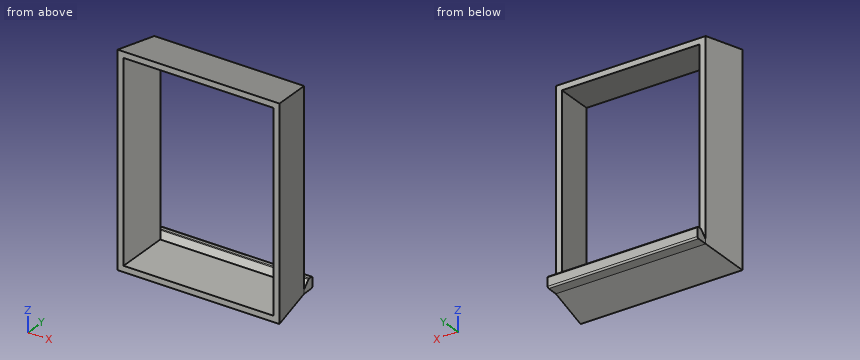
from build123d import *

# Parameters (mm, degrees)
BOSS_EXTRUDE1_DEPTH = 20
LOFT1_START         = -34.8
LOFT1_DEPTH         = 69.6
LOFT1_START_2       = -28
LOFT1_2_DEPTH       = 56
BOSS_EXTRUDE2_START = -2
BOSS_EXTRUDE2_DEPTH = 50
BOSS_EXTRUDE3_DEPTH = 2.3
BOSS_EXTRUDE4_DEPTH = 2.3
CUT_EXTRUDE1_START  = -69.6
SKETCH7_R           = 5.3
CUT_EXTRUDE1_DEPTH  = 2
CUT_EXTRUDE2_DEPTH  = 70
SKETCH9_W           = 56.388818991
SKETCH9_H           = 73.181727467
BOSS_EXTRUDE5_DEPTH = 48


with BuildPart() as part:
    # Sketch1 → Boss-Extrude1 (new body)
    with BuildSketch(Plane(origin=(0, 0, 0), x_dir=(1, 0, 0), z_dir=(0, 1, 0))):
        Polygon((27, 34.8), (-27, 34.8), (-27, 0), (-27, -34.8), (27, -34.8), (27, 0), align=None)
        Polygon((25, 0), (25, 32.8), (-25, 32.8), (-25, 0), (-25, -32.8), (25, -32.8), align=None, mode=Mode.SUBTRACT)
    extrude(amount=BOSS_EXTRUDE1_DEPTH)

    # Loft1: read off the stored shape, not the designer's step
    # Loft1 outline → Loft1 (add)
    with BuildSketch(Plane.XY.offset(LOFT1_START)):
        Polygon((-27, 20), (27, 20), (25, 35), (-25, 35), align=None)
    extrude(amount=LOFT1_DEPTH)

    # Loft1 2 outline → Loft1 2 (cut)
    with BuildSketch(Plane.YZ.offset(LOFT1_START_2)):
        Polygon((20, 34.8), (35, 32.8), (35, 34.8), align=None)
        Polygon((35, -32.8), (20, -34.8), (35, -34.8), align=None)
    extrude(amount=LOFT1_2_DEPTH, mode=Mode.SUBTRACT)

    # Cut-Loft1: read off the stored shape, not the designer's step
    # Cut-Loft1: loft between two sections, ruled curve by curve
    cut_loft1_from = [
        Edge.make_line((-25, 20, 32.8), (-25, 20, -32.8)),
        Edge.make_line((-25, 20, -32.8), (25, 20, -32.8)),
        Edge.make_line((25, 20, 32.8), (-25, 20, 32.8)),
        Edge.make_line((25, 20, -32.8), (25, 20, 32.8)),
    ]
    cut_loft1_to = [
        Edge.make_line((-23, 35, 30.8), (-23, 35, -30.8)),
        Edge.make_line((-23, 35, -30.8), (23, 35, -30.8)),
        Edge.make_line((23, 35, 30.8), (-23, 35, 30.8)),
        Edge.make_line((23, 35, -30.8), (23, 35, 30.8)),
    ]
    cut_loft1 = Solid(Shell([*[Face.make_surface_from_curves(cut_loft1_from[k], cut_loft1_to[k]) for k in range(4)], Face(Wire(cut_loft1_from)), Face(Wire(cut_loft1_to))]))
    add(cut_loft1, mode=Mode.SUBTRACT)

    # Sketch2 → Boss-Extrude2 (add)
    with BuildSketch(Plane(origin=(27, 0, 0), x_dir=(0, 0, -1), z_dir=(1, 0, 0)).offset(BOSS_EXTRUDE2_START)):
        with BuildLine():
            Line((32.8, 35), (32.8, 38.5))
            ThreePointArc((32.8, 38.5), (32.653553391, 38.853553391), (32.3, 39))
            Line((32.3, 39), (29.6, 39))
            ThreePointArc((29.6, 39), (29.246446609, 38.853553391), (29.1, 38.5))
            Line((29.1, 38.5), (29.1, 37.468550682))
            ThreePointArc((29.1, 37.468550682), (29.138060234, 37.277208966), (29.246446609, 37.114997291))
            Line((29.246446609, 37.114997291), (31.361443901, 35))
            Line((31.361443901, 35), (32.8, 35))
        make_face()
    extrude(amount=-BOSS_EXTRUDE2_DEPTH)

    # Sketch7 → Cut-Extrude1 (cut)
    with BuildSketch(Plane.XY.offset(34.8).offset(CUT_EXTRUDE1_START)):
        with Locations((0, 10)):
            Circle(SKETCH7_R)
    extrude(amount=CUT_EXTRUDE1_DEPTH, mode=Mode.SUBTRACT)

    # Sketch8 → Cut-Extrude2 (cut)
    with BuildSketch(Plane.ZY.offset(27)):
        with BuildLine():
            Line((-25.8, 6), (-22.8, 6))
            ThreePointArc((-22.8, 6), (-21.8, 4), (-22.8, 2))
            Line((-22.8, 2), (-25.8, 2))
            ThreePointArc((-25.8, 2), (-26.8, 4), (-25.8, 6))
        make_face()
        with BuildLine():
            Line((22.8, 6), (25.8, 6))
            ThreePointArc((25.8, 6), (26.8, 4), (25.8, 2))
            Line((25.8, 2), (22.8, 2))
            ThreePointArc((22.8, 2), (21.8, 4), (22.8, 6))
        make_face()
    extrude(amount=-CUT_EXTRUDE2_DEPTH, mode=Mode.SUBTRACT)


with BuildPart() as body_2:
    # Sketch5 → Boss-Extrude3 (new body)
    with BuildSketch(Plane.XZ):
        with BuildLine():
            Line((-25, -34.8), (-25, -9.8))
            ThreePointArc((-25, -9.8), (0, 15.2), (25, -9.8))
            Line((25, -9.8), (25, -34.8))
            Line((25, -34.8), (27, -34.8))
            Line((27, -34.8), (27, 34.8))
            Line((27, 34.8), (-27, 34.8))
            Line((-27, 34.8), (-27, -34.8))
            Line((-27, -34.8), (-25, -34.8))
        make_face()
    extrude(amount=BOSS_EXTRUDE3_DEPTH)

    # Sketch6 → Boss-Extrude4 (add)
    with BuildSketch(Plane.XZ.offset(2.3)):
        with BuildLine():
            Line((22.7, -34.8), (27, -34.8))
            Line((27, -34.8), (27, 34.8))
            Line((27, 34.8), (-27, 34.8))
            Line((-27, 34.8), (-27, -34.8))
            Line((-27, -34.8), (-22.7, -34.8))
            Line((-22.7, -34.8), (-22.7, -9.8))
            ThreePointArc((-22.7, -9.8), (0, 12.9), (22.7, -9.8))
            Line((22.7, -9.8), (22.7, -34.8))
        make_face()
    extrude(amount=BOSS_EXTRUDE4_DEPTH)


with BuildPart() as body_2_2:
    # Sketch9 → Boss-Extrude5 (new body)
    with BuildSketch(Plane(origin=(0, 20, 0), x_dir=(-1, 0, 0), z_dir=(0, 1, 0))):
        with Locations((0.397726779, 0.176767457)):
            Rectangle(SKETCH9_W, SKETCH9_H)
    extrude(amount=-BOSS_EXTRUDE5_DEPTH)


with BuildPart() as part_1:
    add(part.part)

    # Combine1: cut body 2 2
    add(body_2_2.part, mode=Mode.SUBTRACT)


solid = part_1.part
Work out the finished part from the listing and answer in its coordinate system (mm). Give positions to 0.01 mm unless a question says otherwise; leave off trailing zeros. Write each loop counter-clockwise with the first axis right and the second up, starting at its lowest first coordinate (ties: lowest second). Pieces come first, ordered by that corner, then holes. Notation, with made-up numbers: (20.5, 62.5) - (38.5, 62.5) arc R17 ccw to (38.5, 95.5) - close; hole circle Ø1 at (-6.5, 6). An arc over 180 degrees is marked (long way). One line per item, written item: value. Start each with the question number.
1. Given pin 1 (0.5 mm diameter, centred on x = 4, y = 38, fed in from +Z); pin 2 (6 mm diameter, centred on y = 27.5, z = 21.5, fed in from +X); pin 3 (5 mm diameter, centred on y = 35.5, z = -11.5, fed in from +X), each flat-ended and moving along its own axis, determine where each tip first touches the part or whether it passes through.
2. Consider probe 1 along X at (y, z) = (32, 7.5); probe 2 along X at (y, z) = (29.25, -5); probe 3 along Z at (x, y) = (-19.5, 31.5). Determine where each line is inside the solid, lowest interval first.
3. Find section A-A (y = 36). Write down the section's boundary in (x, z), then the cut area to 3 significant figures.
Geometry results:
1. pin 1: z = -29.1
1. pin 2: x = 26.4
1. pin 3: x = 25.27
2. probe 1: -25.4 to -23.4, 23.4 to 25.4
2. probe 2: -25.77 to -23.77, 23.77 to 25.77
2. probe 3: -33.27 to -31.27, 31.27 to 33.27
3. outline: (-25, -32.8) - (25, -32.8) - (25, -30.36) - (-25, -30.36) - close
3. area: 122 mm2
